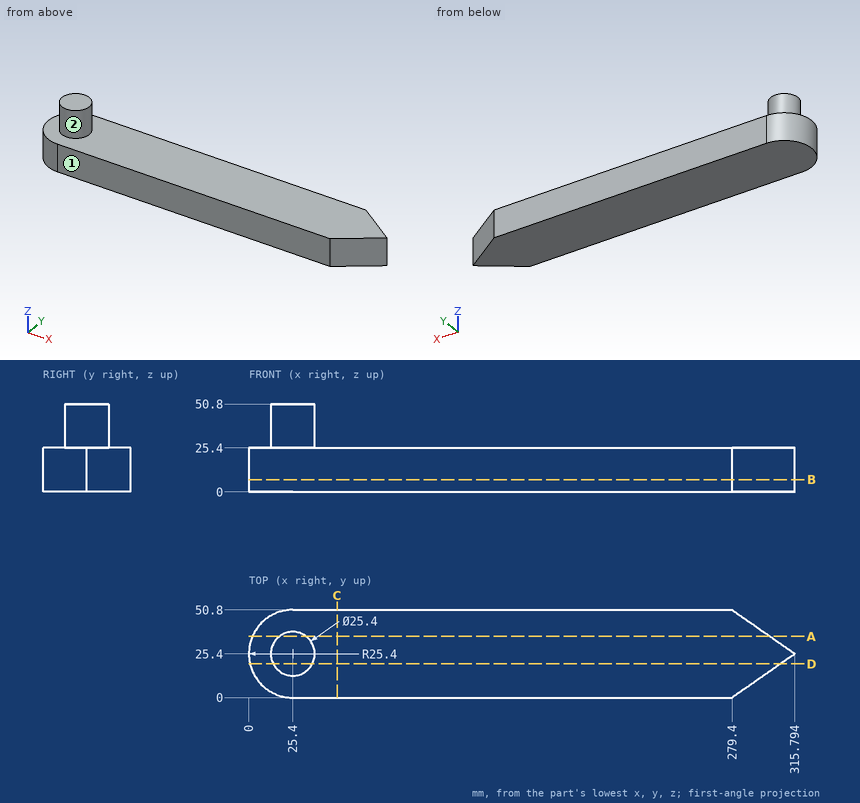
Geometry: see drawing. Coordinates: mm, zero at the bounding-box minimum. A direction names the side the tool comes from. Give positions to 0.01 mm unless a question says otherwise; leave off trailing zeros. Write each loop counter-clockwise with the first axis right and the second up, starting at its lowest first coordinate (ties: lowest second). Pieces come first, ordered by that corner, then holes. Notation, with made-up numbers: (36, -32.5) - (93, -32.5) arc R32 cw to (93, -5.5) - close; hole circle Ø10 at (31.5, -26.75). An arc over 180 degrees is marked (long way). Return JSON: item names as keys, results as strings. Group by question number.
1) Section B-B on z = 7. Return the cut outline in (x, y).
2) Section C-C on x = 51. Return the cut outline in (y, z), plus the area to 3 significant figures.
3) Line query: line 1 (Z direction, x = 212, y = 8); line 2 (X direction, y = 5, z = 18) (1 decimal); line 3 (X direction, y = 29, z = 26.5). Output: solid intervals per line, ascending.
4) Set-up query: the marked faces 1 and 2. Return all of +Z, -Z, +X, -X, +Y, -Y with unobstructed straight access to the full face (end or side cutting, diameter ignored); none if empty.
5) Section A-A on y = 35.5. Return the cut outline in (x, z) (1 decimal).
6) Section D-D on y = 19.5. Return the cut outline in (x, z) (1 decimal).
7) First-contact query: P1, Ø3, axis at y = 34, z = 9, coming from the -X side; P2, Ø2, axis at y = 19.5, z = 7.5, coming from the -X side; P3, Ø6, axis at y = 32.5, z = 10.5, coming from the -X side. Flat tips, straight axial feed; report the tip coordinate or a pass-through.
Filled in:
{
 "1": {"outline": "(25.4, 0) - (279.4, 0) - (315.79, 25.4) - (279.4, 50.8) - (25.4, 50.8) arc R25.4 ccw to start"},
 "2": {"outline": "(0, 0) - (50.8, 0) - (50.8, 25.4) - (0, 25.4) - close", "area": "1,290 mm^2"},
 "3": {"line 1": "z = 0 to 25.4", "line 2": "x = 10.3 to 286.6", "line 3": "x = 13.22 to 37.58"},
 "4": {"face 1": "+Z, -Z, +X, -X, -Y", "face 2": "+Z"},
 "5": {"outline": "(2.1, 0) - (301.3, 0) - (301.3, 25.4) - (33.1, 25.4) - (33.1, 50.8) - (17.7, 50.8) - (17.7, 25.4) - (2.1, 25.4) - close"},
 "6": {"outline": "(0.7, 0) - (307.3, 0) - (307.3, 25.4) - (36.6, 25.4) - (36.6, 50.8) - (14.2, 50.8) - (14.2, 25.4) - (0.7, 25.4) - close"},
 "7": {"P1": "stops at x = 1.01", "P2": "stops at x = 0.48", "P3": "stops at x = 0.33"}
}
